Here's how the part is built. I have some questions about the finished solid (model axes, mm). A direction names the side the tool comes from. Give positions to 0.01 mm unless a question says otherwise; leave off trailing zeros. Order: outer loops, then holes, each group sorted by start corner. A loop starts at its lowest first (then second) coordinate and runs counter-clockwise, first axis right, second up. Notation, with made-up numbers: M 23.25,88 L 45.25,88 A27 cw 45.25,107 Z; hole C 86,71.25 d1. An arc over 180 degrees is marked long. Use one line per item in the form item = value.
from build123d import *

# Parameters (mm, degrees)
SKETCH_1_R      = 55
SKETCH_1_R_2    = 1.5
SKETCH_1_W      = 40
SKETCH_1_H      = 20
EXTRUDE_2_DEPTH = 3


with BuildPart() as part:
    # 草图1 → 凸台-拉伸2 (new body)
    with BuildSketch(Plane.XY):
        Circle(SKETCH_1_R)
        with Locations((-35, 35)):
            Circle(SKETCH_1_R_2, mode=Mode.SUBTRACT)
        with Locations((35, 35)):
            Circle(SKETCH_1_R_2, mode=Mode.SUBTRACT)
        with Locations((35, -35)):
            Circle(SKETCH_1_R_2, mode=Mode.SUBTRACT)
        with Locations((-35, -35)):
            Circle(SKETCH_1_R_2, mode=Mode.SUBTRACT)
        with Locations((-14.3, 5)):
            Circle(SKETCH_1_R_2, mode=Mode.SUBTRACT)
        with Locations((-14.3, -5)):
            Circle(SKETCH_1_R_2, mode=Mode.SUBTRACT)
        with Locations((34.3, 5)):
            Circle(SKETCH_1_R_2, mode=Mode.SUBTRACT)
        with Locations((34.3, -5)):
            Circle(SKETCH_1_R_2, mode=Mode.SUBTRACT)
        with Locations((10, 0)):
            Rectangle(SKETCH_1_W, SKETCH_1_H, mode=Mode.SUBTRACT)
    extrude(amount=EXTRUDE_2_DEPTH)


solid = part.part
Q1. I want a section at A-A on y = 0. Write out the boundary of the cut face in (x, z).
Found:
outline = M -55,0 L -10,0 L -10,3 L -55,3 Z; M 30,0 L 55,0 L 55,3 L 30,3 Z
Q2. I need wall thicknesses on L1, parallel to Y at x = -14.3, z = 2.05; L2, parallel to Y at x = 34.3, z = 1.35; L3, parallel to X at y = 36, z = 1.5. Which ranges of each line are inside material? Lowest first, please.
Found:
L1 = -53.11 to -6.5, -3.5 to 3.5, 6.5 to 53.11
L2 = -42.99 to -36.33, -33.67 to -6.5, -3.5 to 3.5, 6.5 to 33.67, 36.33 to 42.99
L3 = -41.58 to -36.12, -33.88 to 33.88, 36.12 to 41.58
Q3. I want a section at B-B on z = 1.5. State how many separate pieces and enclosed holes the cut face has, then the cut area to 3 significant figures.
Found:
separate_pieces = 1
enclosed_holes = 9
area = 8,650 mm²
Q4. I'm going to push flat-ended pins straight in: pin 1 Ø1.5 at (x, z) = (16, 1.5) entering from +Y; pin 2 Ø1.8 at (x, y) = (35, 35) entering from +Z. Where does each tip first touch, or does it pass through?
Found:
pin_1 = 52.84
pin_2 = through
Q5. On a 3-axis mill with a long thin cutter (end or side, diameter ignored), from which of +Z, -Z, +X, -X, +Y, -Y can I reach the whole of each face in a straight line? I mean faces 4 (the face through (-1, -11, 0)), 5 (the face through (10, 10, 1)). Say none if no direction works.
Found:
face_4 = -Z, +X, -X, +Y, -Y
face_5 = +Z, -Z
Q6. I want a section at C-C on x = 0. Write out the boundary of the cut face in (y, z).
Found:
outline = M -55,0 L -10,0 L -10,3 L -55,3 Z; M 10,0 L 55,0 L 55,3 L 10,3 Z
Q7. Thinking about a two-plate mould opening in Y: for faces 1 (the face through (-1, -11, 3)), 2 (the face through (30, 0, 1)), 3 (the face through (-11.923, -53.692, 1.479)), which applies, +Y half, -Y half, draft (parallel to the pull), parting line (faces both ways), or undercut?
Found:
face_1 = draft
face_2 = undercut
face_3 = parting line
Q8. I want a section at D-D on x = -14.3. Write out the boundary of the cut face in (y, z).
Found:
outline = M -53.11,0 L -6.5,0 L -6.5,3 L -53.11,3 Z; M -3.5,0 L 3.5,0 L 3.5,3 L -3.5,3 Z; M 6.5,0 L 53.11,0 L 53.11,3 L 6.5,3 Z
